```python
from build123d import *

# Parameters (mm, degrees)
F1_DEPTH  = 339.7
F2_R      = 7.95
F3_R      = 7.95
F4_R      = 48.895
F5_DEPTH  = 9.526
F6_D      = 8.4328
F8_D      = 26
F8_DEPTH  = 63.008
F9_R      = 19.05
F10_DEPTH = 25


with BuildPart() as f1:
    # F0 (on Front) → F1 (new body)
    with BuildSketch(Plane.XZ):
        with BuildLine():
            Line((0, -267.168), (0, 0))
            Line((0, 0), (-9.525, 0))
            Line((-9.525, 0), (-9.525, -267.168))
            ThreePointArc((-9.525, -267.168), (-3.9453841816, -280.6383841816), (9.525, -286.218))
            Line((9.525, -286.218), (68.513, -286.218))
            Line((68.513, -286.218), (68.513, -339.7))
            Line((68.513, -339.7), (78.038, -339.7))
            Line((78.038, -339.7), (78.038, -276.693))
            Line((78.038, -276.693), (9.525, -276.693))
            ThreePointArc((9.525, -276.693), (2.7898079092, -273.9031920908), (0, -267.168))
        make_face()
    extrude(amount=F1_DEPTH)

    # F2
    f2_edges = [f1.edges().sort_by_distance(p)[0] for p in [
        (-4.7625, -339.7, 0),
    ]]
    fillet(f2_edges, radius=F2_R)

    # F3
    f3_edges = [f1.edges().sort_by_distance(p)[0] for p in [
        (-4.7625, 0, 0),
        (73.2755, 0, -339.7),
        (73.2755, -339.7, -339.7),
    ]]
    fillet(f3_edges, radius=F3_R)

    # F4 (on face) → F5 (cut, through all)
    with BuildSketch(Plane.YZ):
        with Locations((-76.541, -139.04)):
            Circle(F4_R)
        with Locations((-263.83, -139.04)):
            Circle(F4_R)
    extrude(amount=-F5_DEPTH, mode=Mode.SUBTRACT)

    # F6 (through all)
    with Locations(Plane.YZ):
        with Locations((-263.83, -81.89), (-313.3233518263, -110.465), (-313.3233518263, -167.615), (-263.83, -196.19), (-214.3366481737, -167.615), (-214.3366481737, -110.465), (-126.0343518263, -110.465), (-76.541, -81.89), (-27.0476481737, -110.465), (-27.0476481737, -167.615), (-76.541, -196.19), (-126.0343518263, -167.615)):
            Hole(F6_D / 2)

    # F8 (through all, one way)
    with BuildSketch(Plane.XY.offset(-276.693)):
        with Locations((20.238, -30.665), (20.238, -121.745), (20.238, -217.955), (20.238, -309.035)):
            Circle(F8_D / 2)
    extrude(amount=-F8_DEPTH, mode=Mode.SUBTRACT)

    # F9 (on face) → F10 (cut)
    with BuildSketch(Plane.XY.offset(-276.693)):
        with Locations((20.238, -30.665)):
            Circle(F9_R)
        with Locations((20.238, -121.745)):
            Circle(F9_R)
        with Locations((20.238, -217.955)):
            Circle(F9_R)
        with Locations((20.238, -309.035)):
            Circle(F9_R)
    extrude(amount=F10_DEPTH, mode=Mode.SUBTRACT)


solid = f1.part
```
For this review, take the finished solid that the model builds, in its own axes (mm). A direction names the side the tool comes from. Give positions to 0.01 mm unless a question says otherwise; leave off trailing zeros. Loops run counter-clockwise (first coordinate to the right, second up) from the corner with the lowest first, then second, coordinate; pieces in that order, holes last. Notation, with made-up numbers: M -36.5,50 L -28.5,50 A20 ccw -28.5,67 Z; hole C 29.25,7 d1. An arc over 180 degrees is marked long. One line per item, written item: value. Start each with the question number.
Q1. Clearance check with flat-ended pins moving along their axes: pin 1 Ø7.5 at (y, z) = (-76.541, -196.19) entering from -X; pin 2 Ø10 at (x, y) = (56.5, -77.5) entering from -Z; pin 3 Ø9.5 at (y, z) = (-214.34, -167.62) entering from +X; pin 4 Ø5 at (x, y) = (66.5, -249.5) entering from -Z. State where each tip first meets the part, or that it passes through.
Q2. Draft analysis for pull direction Y (two halves, no side actions). For faces 1 (the face through (-2, -339.7, -193)), 2 (the face through (-4.829, -125.485, -163.434)), 3 (the face through (-9.525, -167, -132)), 4 (the face through (-4.8, -211.2, -164.8)), state which applies: released by +Y, released by -Y, zero draft, split by the parting line, or undercut.
Q3. For L1, parallel to Y at x = -6, z = -81; L2, parallel to Y at x = -1, z = -196.5; L3, parallel to Z at x = 45.5, y = -324, list the stretches that pass through material, from the lowest coordinate up.
Q4. Machinability: for faces 5 (the face through (17.42, -230.646, -281.389)), 6 (the face through (1.19, -30.41, -274.81)), which of the approach directions +Z, -Z, +X, -X, +Y, -Y give a long, thin tool a straight path to every point of the face, cutting with its end or side? Answer none if there is none.
Q5. Add section B-B (z = -196.19). Give the boundary of the cut face in (x, y) (3 decimals).
Q6. Add section D-D (y = -155). Give the boundary of the cut face in (x, z) (3 decimals), and give its area (3 significant figures).
Q7. Add section C-C (z = -139.04). Give the boundary of the cut face in (x, y) (3 decimals), and give its area (3 significant figures).
Q8. Add section A-A (y = -263.83). Give the boundary of the cut face in (x, z) (3 decimals), and give its area (3 significant figures).
Reply:
1. pin 1: through
1. pin 2: z = -286.22
1. pin 3: x = 0
1. pin 4: z = -339.7
2. face 1: released by -Y
2. face 2: undercut
2. face 3: zero draft
2. face 4: undercut
3. L1: -339.7 to -267.95, -259.71 to -80.66, -72.42 to 0
3. L2: -339.7 to -268.03, -259.63 to -80.75, -72.34 to 0
3. L3: -286.22 to -276.69
4. face 5: +Z, -Z
4. face 6: +Z, +X
5. outline: M -9.525,-339.7 L 0,-339.7 L 0,-268.046 L -9.525,-268.046 Z; M -9.525,-259.614 L 0,-259.614 L 0,-80.757 L -9.525,-80.757 Z; M -9.525,-72.325 L 0,-72.325 L 0,0 L -9.525,0 Z
6. outline: M -9.525,-267.168 A19.05 ccw 9.525,-286.218 L 68.513,-286.218 L 68.513,-339.7 L 78.038,-339.7 L 78.038,-276.693 L 9.525,-276.693 A9.525 cw 0,-267.168 L 0,0 L -9.525,0 Z
6. area: 3,920 mm²
7. outline: M -9.525,-339.7 L 0,-339.7 L 0,-312.725 L -9.525,-312.725 Z; M -9.525,-214.935 L 0,-214.935 L 0,-125.436 L -9.525,-125.436 Z; M -9.525,-27.646 L 0,-27.646 L 0,0 L -9.525,0 Z
7. area: 1,370 mm²
8. outline: M -9.525,-267.168 A19.05 ccw 9.525,-286.218 L 68.513,-286.218 L 68.513,-339.7 L 78.038,-339.7 L 78.038,-276.693 L 9.525,-276.693 A9.525 cw 0,-267.168 L 0,-200.406 L -9.525,-200.406 Z; M -9.525,-191.974 L 0,-191.974 L 0,-187.935 L -9.525,-187.935 Z; M -9.525,-90.145 L 0,-90.145 L 0,-86.106 L -9.525,-86.106 Z; M -9.525,-77.674 L 0,-77.674 L 0,0 L -9.525,0 Z
8. area: 2,830 mm²
